from build123d import *

# Parameters (mm, degrees)
EXTRUDE_1_DEPTH     = 50
SKETCH_2_R          = 5
CUT_EXTRUDE_1_DEPTH = 10


with BuildPart() as part:
    # Эскиз1 → Вытянуть-Тонкостенный1 (new body)
    with BuildSketch(Plane.XY):
        Polygon((0, 30), (0, 0), (30, 0), (30, -3), (-3, -3), (-3, 30), align=None)
    extrude(amount=-EXTRUDE_1_DEPTH)

    # Эскиз2 → Вырез-Вытянуть1 (cut)
    with BuildSketch(Plane.ZX.offset(-3)):
        with Locations(Location((-40, 15, 0), (0, 0, 180))):
            Circle(SKETCH_2_R)
    extrude(amount=CUT_EXTRUDE_1_DEPTH, mode=Mode.SUBTRACT)


solid = part.part
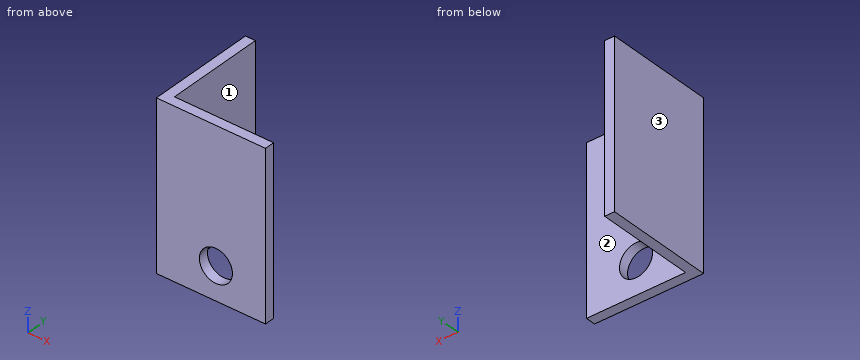
Geometry: final body of the model. Coordinates: model frame, mm. Face numbers are marked on the shaded views. Give positions to 0.01 mm unless a question says otherwise; leave off trailing zeros. Write each loop counter-clockwise with the first axis right and the second up, starting at its lowest first coordinate (ties: lowest second). Pieces come first, ordered by that corner, then holes.
(1) Cut plane C-C, the plane z = -4.5. Return loops of the section in (x, y).
(2) Cut plane D-D, the plane y = 14. Return loops of the section in (x, z).
(3) Ray query, line 1 (X direction, y = -0.8, z = -40); line 2 (Z direction, x = 15, y = -0.95); line 3 (Y direction, x = 9, z = -33). Return the intervals inside material, ascending.
(4) Mould query, pull axis X, two halves, no side actions, for the marked faces 1, 2 and 3. Classes: released by +X, released by -X, zero draft, split by the parting line, or undercut.
(5) Cut plane B-B, the plane x = 15. Return loops of the section in (y, z), then the cut area to 3 significant figures.
(6) First-contact query: P1, Ø4, axis at y = 9.5, z = -32, coming from the +X side; P2, Ø9, axis at x = 15, z = -40, coming from the +Y side; P3, Ø10, axis at x = 7.5, z = -37, coming from the +Y side. Flat tips, straight axial feed; report the tip coordinate or a pass-through.
(7) Cut plane A-A, the plane z = -40. Return loops of the section in (x, y).
Values follow:
1. outline: (-3, -3) - (30, -3) - (30, 0) - (0, 0) - (0, 30) - (-3, 30) - close
2. outline: (-3, -50) - (0, -50) - (0, 0) - (-3, 0) - close
3. line 1: x = -3 to 10, 20 to 30
3. line 2: z = -50 to -45, -35 to 0
3. line 3: y = -3 to 0
4. face 1: released by +X
4. face 2: zero draft
4. face 3: released by -X
5. outline: (-3, -50) - (0, -50) - (0, -45) - (-3, -45) - close; (-3, -35) - (0, -35) - (0, 0) - (-3, 0) - close
5. area: 120 mm2
6. P1: stops at x = 0
6. P2: passes through
6. P3: stops at y = 0
7. outline: (-3, -3) - (10, -3) - (10, 0) - (0, 0) - (0, 30) - (-3, 30) - close; (20, -3) - (30, -3) - (30, 0) - (20, 0) - close
